from build123d import *

# Parameters (mm, degrees)
SKETCH_1_W                         = 2.79
SKETCH_1_H                         = 5
EXTRUDE_1_DEPTH                    = 8.4
SKETCH_2_W                         = 1
SKETCH_2_H                         = 1
CUT_EXTRUDE_1_DEPTH                = 8
CHAMFER_1_SIZE                     = 0.2
SKETCH_3_W                         = 0.64
SKETCH_3_H                         = 0.64
EXTRUDE_2_DEPTH                    = 2.29
CHAMFER_2_SIZE                     = 0.2
PATTERN_LINEAR_1_COUNT             = 6
PATTERN_LINEAR_1_PITCH             = 2.54
CHAMFER_1_OF_PATTERN_LINEAR_1_SIZE = 0.2
CHAMFER_2_OF_PATTERN_LINEAR_1_SIZE = 0.2


with BuildPart() as part:
    # Эскиз1 → Бобышка-Вытянуть1 (new body)
    with BuildSketch(Plane(origin=(0, 0, 0), x_dir=(1, 0, 0), z_dir=(0, 1, 0))):
        Rectangle(SKETCH_1_W, SKETCH_1_H)
    extrude_1 = extrude(amount=EXTRUDE_1_DEPTH)

    # Эскиз2 → Вырез-Вытянуть1 (cut)
    with BuildSketch(Plane(origin=(0, 8.4, 0), x_dir=(1, 0, 0), z_dir=(0, 1, 0))):
        with Locations((0, 1.27)):
            Rectangle(SKETCH_2_W, SKETCH_2_H)
        with Locations((0, -1.27)):
            Rectangle(SKETCH_2_W, SKETCH_2_H)
    cut_extrude_1 = extrude(amount=-CUT_EXTRUDE_1_DEPTH, mode=Mode.SUBTRACT)

    # Фаска1
    chamfer_1_edges = [part.edges().sort_by_distance(p)[0] for p in [
        (0.5, 8.4, -1.27),
        (0, 8.4, -1.77),
        (-0.5, 8.4, -1.27),
        (0, 8.4, -0.77),
        (0, 8.4, 1.77),
        (0.5, 8.4, 1.27),
        (0, 8.4, 0.77),
        (-0.5, 8.4, 1.27),
    ]]
    chamfer(chamfer_1_edges, length=CHAMFER_1_SIZE)

    # Эскиз3 → Бобышка-Вытянуть2 (add)
    with BuildSketch(Plane(origin=(0, 0, 0), x_dir=(-1, 0, 0), z_dir=(0, -1, 0))):
        with Locations((0, 1.27)):
            Rectangle(SKETCH_3_W, SKETCH_3_H)
        with Locations((0, -1.27)):
            Rectangle(SKETCH_3_W, SKETCH_3_H)
    extrude_2 = extrude(amount=EXTRUDE_2_DEPTH)

    # Фаска2
    chamfer_2_edges = [part.edges().sort_by_distance(p)[0] for p in [
        (0.32, -2.29, -1.27),
        (0, -2.29, -0.95),
        (-0.32, -2.29, -1.27),
        (0, -2.29, -1.59),
        (-0.32, -2.29, 1.27),
        (0, -2.29, 0.95),
        (0.32, -2.29, 1.27),
        (0, -2.29, 1.59),
    ]]
    chamfer(chamfer_2_edges, length=CHAMFER_2_SIZE)

    # Линейный массив1: Бобышка-Вытянуть1, Вырез-Вытянуть1, Бобышка-Вытянуть2 ×6
    with Locations(*[(i * PATTERN_LINEAR_1_PITCH, 0, 0) for i in range(1, PATTERN_LINEAR_1_COUNT)]):
        add(extrude_1)
        add(cut_extrude_1, mode=Mode.SUBTRACT)
        add(extrude_2)

    # Фаска1 of Линейный массив1
    chamfer_1_of_pattern_linear_1_edges = [part.edges().sort_by_distance(p)[0] for p in [
        (3.04, 8.4, -1.27),
        (2.54, 8.4, -1.77),
        (2.04, 8.4, -1.27),
        (2.54, 8.4, -0.77),
        (2.54, 8.4, 1.77),
        (3.04, 8.4, 1.27),
        (2.54, 8.4, 0.77),
        (2.04, 8.4, 1.27),
        (5.58, 8.4, -1.27),
        (5.08, 8.4, -1.77),
        (4.58, 8.4, -1.27),
        (5.08, 8.4, -0.77),
        (5.08, 8.4, 1.77),
        (5.58, 8.4, 1.27),
        (5.08, 8.4, 0.77),
        (4.58, 8.4, 1.27),
        (8.12, 8.4, -1.27),
        (7.62, 8.4, -1.77),
        (7.12, 8.4, -1.27),
        (7.62, 8.4, -0.77),
        (7.62, 8.4, 1.77),
        (8.12, 8.4, 1.27),
        (7.62, 8.4, 0.77),
        (7.12, 8.4, 1.27),
        (10.66, 8.4, -1.27),
        (10.16, 8.4, -1.77),
        (9.66, 8.4, -1.27),
        (10.16, 8.4, -0.77),
        (10.16, 8.4, 1.77),
        (10.66, 8.4, 1.27),
        (10.16, 8.4, 0.77),
        (9.66, 8.4, 1.27),
        (13.2, 8.4, -1.27),
        (12.7, 8.4, -1.77),
        (12.2, 8.4, -1.27),
        (12.7, 8.4, -0.77),
        (12.7, 8.4, 1.77),
        (13.2, 8.4, 1.27),
        (12.7, 8.4, 0.77),
        (12.2, 8.4, 1.27),
    ]]
    chamfer(chamfer_1_of_pattern_linear_1_edges, length=CHAMFER_1_OF_PATTERN_LINEAR_1_SIZE)

    # Фаска2 of Линейный массив1
    chamfer_2_of_pattern_linear_1_edges = [part.edges().sort_by_distance(p)[0] for p in [
        (2.86, -2.29, -1.27),
        (2.54, -2.29, -0.95),
        (2.22, -2.29, -1.27),
        (2.54, -2.29, -1.59),
        (2.22, -2.29, 1.27),
        (2.54, -2.29, 0.95),
        (2.86, -2.29, 1.27),
        (2.54, -2.29, 1.59),
        (5.4, -2.29, -1.27),
        (5.08, -2.29, -0.95),
        (4.76, -2.29, -1.27),
        (5.08, -2.29, -1.59),
        (4.76, -2.29, 1.27),
        (5.08, -2.29, 0.95),
        (5.4, -2.29, 1.27),
        (5.08, -2.29, 1.59),
        (7.94, -2.29, -1.27),
        (7.62, -2.29, -0.95),
        (7.3, -2.29, -1.27),
        (7.62, -2.29, -1.59),
        (7.3, -2.29, 1.27),
        (7.62, -2.29, 0.95),
        (7.94, -2.29, 1.27),
        (7.62, -2.29, 1.59),
        (10.48, -2.29, -1.27),
        (10.16, -2.29, -0.95),
        (9.84, -2.29, -1.27),
        (10.16, -2.29, -1.59),
        (9.84, -2.29, 1.27),
        (10.16, -2.29, 0.95),
        (10.48, -2.29, 1.27),
        (10.16, -2.29, 1.59),
        (13.02, -2.29, -1.27),
        (12.7, -2.29, -0.95),
        (12.38, -2.29, -1.27),
        (12.7, -2.29, -1.59),
        (12.38, -2.29, 1.27),
        (12.7, -2.29, 0.95),
        (13.02, -2.29, 1.27),
        (12.7, -2.29, 1.59),
    ]]
    chamfer(chamfer_2_of_pattern_linear_1_edges, length=CHAMFER_2_OF_PATTERN_LINEAR_1_SIZE)


solid = part.part
Input: part model. Units: mm. Frame: model coordinates. Coordinates: 2 decimals unless noted, no trailing zeros. Loops run counter-clockwise (first coordinate to the right, second up) from the corner with the lowest first, then second, coordinate; pieces in that order, holes last. Notation, with made-up numbers: (-29.75, 89) - (-24.75, 89) arc R31 ccw to (-24.75, 114) - close; hole circle Ø3 at (27, 27). An arc over 180 degrees is marked (long way). Answer in a Markdown table with one row per item. Add a question column.
Item 1: Section query C-C on z = 0. Return the cut outline in (x, y) (3 decimals), then the cut area to 3 significant figures.
Item 2: Mould query, pull axis Z, two halves, no side actions, for faces 1 (the flat face through (12.2, 4, 1)), 2 (the flat face through (-1.395, 4, 0)). Classes: released by +Z, released by -Z, zero draft, split by the parting line, or undercut.
Item 3: Section query A-A on y = -0.5. State how many separate pieces and enclosed holes the cut face has, then the cut area to 3 significant figures.
Item 4: Contact query for a flat-ended pin moving along its axis: P1, Ø1.1, axis at x = 10.5, z = 1, coming from the +Y side. Output: stop coordinate, or through.
Item 5: Line query: line 1 along Z through (x, y) = (5.5, 1); line 2 along X through (y, z) = (-0.5, 1); line 3 along Y through (x, z) = (9.25, -0.85). Output: solid intervals per line, ascending. Write a range as [from, to].
Recorded:
| question | item | result |
|---|---|---|
| 1 | outline | (-1.395, 0) - (14.095, 0) - (14.095, 8.4) - (-1.395, 8.4) - close |
| 1 | area | 130 mm^2 |
| 2 | face 1 | undercut |
| 2 | face 2 | zero draft |
| 3 | separate pieces | 12 |
| 3 | enclosed holes | 0 |
| 3 | area | 4.92 mm^2 |
| 4 | P1 | y = 8.4 |
| 5 | line 1 | [-2.5, -1.77], [-0.77, 0.77], [1.77, 2.5] |
| 5 | line 2 | [-0.32, 0.32], [2.22, 2.86], [4.76, 5.4], [7.3, 7.94], [9.84, 10.48], [12.38, 13.02] |
| 5 | line 3 | [0, 8.4] |
